The listing builds one solid part. Answer for the finished solid, in the listing's coordinates (mm). Face numbers are marked on the shaded views. A direction names the side the tool comes from. Round coordinates to 2 decimals unless told otherwise and drop trailing zeros. Write each loop counter-clockwise with the first axis right and the second up, starting at its lowest first coordinate (ties: lowest second). Pieces come first, ordered by that corner, then holes. Notation, with made-up numbers: (62.5, -25) - (96.5, -25) arc R27 cw to (96.5, -2) - close; hole circle Ø8 at (66, -34.5). An arc over 180 degrees is marked (long way). Answer as CSV lines item,"result". Start each with the question number.
Item 1: A cutting plane is placed at A-A on z = 300. Determine the outline of the cut face in (x, y).
Item 2: Flat-ended cylindrical pins translate along their axes: pin 1 (6.5 mm diameter, centred on x = 241.5, z = 269, fed in from -Y); pin 2 (5 mm diameter, centred on x = 238, y = 290.5, fed in from -Z); pin 3 (10 mm diameter, centred on y = 279.5, z = 311, fed in from +X); pin 4 (1 mm diameter, centred on x = 226.5, z = 302.5, fed in from -Y). Find the tip coordinate at first contact, or state that the pin passes through.
Item 3: A cutting plane is placed at B-B on x = 238. Determine the outline of the cut face in (y, z).
Item 4: A cutting plane is placed at D-D on z = 292. Determine the outline of the cut face in (x, y).
Item 5: Which of the six approach directions +Z, -Z, +X, -X, +Y, -Y give full straight-line access (tool end or side, diameter ignored) to the marked faces 4, 5 and 6?
Item 6: A cutting plane is placed at C-C on y = 292. Determine the outline of the cut face in (x, z), and give its area (3 significant figures).
Item 7: Straight lines are drawn through the part: line 1 along Y through (x, z) = (224.7, 300); line 2 along Y through (x, z) = (238, 262.35); line 3 along Z through (x, y) = (243.5, 283.5). For each, find the intervals that lie inside material, in ascending order. Write a range as [from, to].
Item 8: For a pull along Y with two mould halves and no side action, classify the marked faces 1, 2 and 3 as pulls with the +Y half, pulls with the -Y half, needs draft (parallel to the pull), parting line crosses it, or undercut.
```python
from build123d import *

# Parameters (mm, degrees)
SKETCH1_R           = 27
BOSS_EXTRUDE1_DEPTH = 6
SKETCH2_W           = 25
SKETCH2_H           = 40
BOSS_EXTRUDE2_DEPTH = 6
SKETCH3_R           = 10
SKETCH3_R_2         = 1.45
CUT_EXTRUDE1_DEPTH  = 6
SKETCH4_W           = 22.01
SKETCH4_H           = 40
SKETCH4_R           = 2.75
BOSS_EXTRUDE3_DEPTH = 6


with BuildPart() as part:
    # Sketch1 → Boss-Extrude1 (new body)
    with BuildSketch(Plane(origin=(221, 0, 0), x_dir=(0, 0, -1), z_dir=(1, 0, 0))):
        with Locations((-300, 300)):
            Circle(SKETCH1_R)
    extrude(amount=BOSS_EXTRUDE1_DEPTH)

    # Sketch2 → Boss-Extrude2 (add)
    with BuildSketch(Plane(origin=(221, 0, 0), x_dir=(0, 0, -1), z_dir=(1, 0, 0))):
        with Locations((-272.5, 300)):
            Rectangle(SKETCH2_W, SKETCH2_H)
    extrude(amount=BOSS_EXTRUDE2_DEPTH)

    # Sketch3 → Cut-Extrude1 (cut)
    with BuildSketch(Plane(origin=(221, 0, 0), x_dir=(0, 0, -1), z_dir=(1, 0, 0))):
        with Locations((-300, 300)):
            Circle(SKETCH3_R)
        with Locations((-300, 322.5)):
            Circle(SKETCH3_R_2)
        with Locations((-278.601228383, 306.952882373)):
            Circle(SKETCH3_R_2)
        with Locations((-286.774831823, 281.797117627)):
            Circle(SKETCH3_R_2)
        with Locations((-313.225168177, 281.797117627)):
            Circle(SKETCH3_R_2)
        with Locations((-321.398771617, 306.952882373)):
            Circle(SKETCH3_R_2)
    extrude(amount=CUT_EXTRUDE1_DEPTH, mode=Mode.SUBTRACT)

    # Sketch4 → Boss-Extrude3 (add)
    with BuildSketch(Plane.XY.offset(260)):
        with Locations((237.995, 300)):
            Rectangle(SKETCH4_W, SKETCH4_H)
        with Locations((238, 290.5)):
            Circle(SKETCH4_R, mode=Mode.SUBTRACT)
        with Locations((238, 309.5)):
            Circle(SKETCH4_R, mode=Mode.SUBTRACT)
    extrude(amount=BOSS_EXTRUDE3_DEPTH)


solid = part.part
```
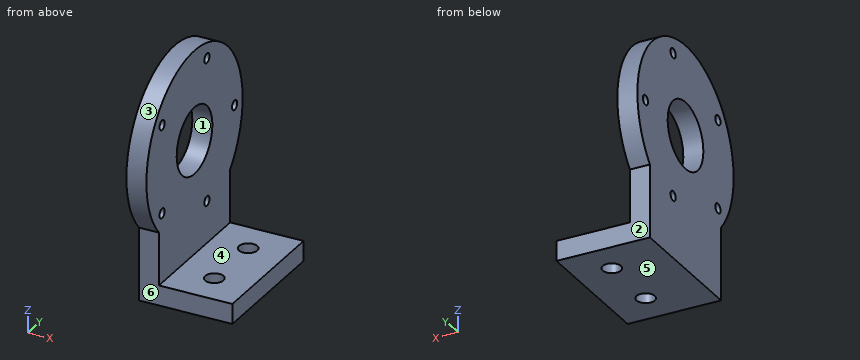
Geometry says:
1,outline,"(221, 273) - (227, 273) - (227, 290) - (221, 290) - close; (221, 310) - (227, 310) - (227, 321.05) - (221, 321.05) - close; (221, 323.95) - (227, 323.95) - (227, 327) - (221, 327) - close"
2,pin 1,"stops at y = 280"
2,pin 2,"passes through"
2,pin 3,"stops at x = 227"
2,pin 4,"stops at y = 273.07"
3,outline,"(280, 260) - (287.75, 260) - (287.75, 266) - (280, 266) - close; (293.25, 260) - (306.75, 260) - (306.75, 266) - (293.25, 266) - close; (312.25, 260) - (320, 260) - (320, 266) - (312.25, 266) - close"
4,outline,"(221, 274.21) - (227, 274.21) - (227, 294) - (221, 294) - close; (221, 306) - (227, 306) - (227, 325.79) - (221, 325.79) - close"
5,face 4,"+Z, +X, +Y, -Y"
5,face 5,"-Z, +X, -X, +Y, -Y"
5,face 6,"-Z, +X, -X, -Y"
6,outline,"(221, 260) - (235.7, 260) - (235.7, 266) - (227, 266) - (227, 294) - (221, 294) - close; (221, 306) - (227, 306) - (227, 325.79) - (221, 325.79) - close; (240.3, 260) - (249, 260) - (249, 266) - (240.3, 266) - close"
6,area,"427 mm^2"
7,line 1,"y = [273, 290], [310, 321.05], [323.95, 327]"
7,line 2,"y = [280, 287.75], [293.25, 306.75], [312.25, 320]"
7,line 3,"z = [260, 266]"
8,face 1,"undercut"
8,face 2,"pulls with the +Y half"
8,face 3,"parting line crosses it"
